Can you work these out from the model? Positions are in its coordinate system, mm. Give positions to 0.01 mm unless a question says otherwise; leave off trailing zeros. Write each loop counter-clockwise with the first axis right and the second up, starting at its lowest first coordinate (ties: lowest second). Pieces come first, ordered by that corner, then holes.
1. Suppose I cut it at A-A (y = -6). Please give me the cut outline in (x, z), and give its area (3 significant figures).
2. Suppose I cut it at B-B (z = 0.3). Please give me the cut outline in (x, y).
3. Suppose I cut it at C-C (x = -50.5). Please give me the cut outline in (y, z).
4. If I drill on probe 1 along X at (y, z) = (-18, 0.55); probe 2 along Y at (x, z) = (-57, 0.9); probe 3 along X at (y, z) = (23, 0.3), over which ranges is the centre line in solid material (lowest first)?
```python
from build123d import *

# Parameters (mm, degrees)
SKETCH_1_W          = 240
SKETCH_1_H          = 50
EXTRUDE_1_DEPTH     = 1
FILLET_1_R          = 3
SKETCH_2_W          = 10
SKETCH_2_H          = 22
CUT_EXTRUDE_1_DEPTH = 123.580585739


with BuildPart() as part:
    # 草图1 → 凸台-拉伸1 (new body)
    with BuildSketch(Plane.XY):
        Rectangle(SKETCH_1_W, SKETCH_1_H)
    extrude(amount=EXTRUDE_1_DEPTH)

    # 圆角1
    fillet_1_edges = [part.edges().sort_by_distance(p)[0] for p in [
        (120, -25, 0.5),
        (-120, -25, 0.5),
        (-120, 25, 0.5),
        (120, 25, 0.5),
    ]]
    fillet(fillet_1_edges, radius=FILLET_1_R)

    # 草图2 → 切除-拉伸1 (cut, through all)
    with BuildSketch(Plane.XY.offset(1)):
        with Locations((-52.5, -14)):
            Rectangle(SKETCH_2_W, SKETCH_2_H)
        with Locations((52.5, -14)):
            Rectangle(SKETCH_2_W, SKETCH_2_H)
    extrude(amount=-CUT_EXTRUDE_1_DEPTH, mode=Mode.SUBTRACT)


solid = part.part
```
Checks:
1. outline: (-120, 0) - (-57.5, 0) - (-57.5, 1) - (-120, 1) - close; (-47.5, 0) - (47.5, 0) - (47.5, 1) - (-47.5, 1) - close; (57.5, 0) - (120, 0) - (120, 1) - (57.5, 1) - close
1. area: 220 mm2
2. outline: (-120, -22) arc R3 ccw to (-117, -25) - (-57.5, -25) - (-57.5, -3) - (-47.5, -3) - (-47.5, -25) - (47.5, -25) - (47.5, -3) - (57.5, -3) - (57.5, -25) - (117, -25) arc R3 ccw to (120, -22) - (120, 22) arc R3 ccw to (117, 25) - (-117, 25) arc R3 ccw to (-120, 22) - close
3. outline: (-3, 0) - (25, 0) - (25, 1) - (-3, 1) - close
4. probe 1: x = -120 to -57.5, -47.5 to 47.5, 57.5 to 120
4. probe 2: y = -3 to 25
4. probe 3: x = -119.83 to 119.83
